Verification items for the finished model (mm, model axes). Face numbers are marked on the shaded views. A direction names the side the tool comes from. Give positions to 0.01 mm unless a question says otherwise; leave off trailing zeros. Write each loop counter-clockwise with the first axis right and the second up, starting at its lowest first coordinate (ties: lowest second). Pieces come first, ordered by that corner, then holes. Notation, with made-up numbers: (-1.5, 52) -> (17.5, 52) arc R3 cw to (17.5, 57) -> close; hole circle Ø1 at (-29.5, 65). An arc over 180 degrees is marked (long way). Answer as CSV lines item,"result". Start each with the question number.
1) Sectioned sample at B-B on z = 0. Record the cut outline in (x, y) (3 decimals), and give its area (3 significant figures).
2) Tool access check on the marked faces 1, 2 and 3. Record the directions out of +Z, -Z, +X, -X, +Y, -Y that give a thin tool (end or side, any length) a straight path to the whole face; none if there is none.
3) Mould release check, pull along X, two halves, no side actions. Record for the marked faces 4, 5 and 6: released by +X, released by -X, zero draft, split by the parting line, or undercut.
4) Sectioned sample at A-A on x = 0. Record the cut outline in (y, z) (3 decimals), and give its area (3 significant figures).
5) Sectioned sample at C-C on z = -9. Record the cut outline in (x, y).
6) Material ranges on L1, parallel to X at y = 0.7, z = 0 (3 decimals); L2, parallel to X at y = 3.25, z = 0 (3 decimals); L3, parallel to Z at x = 3.5, y = 3.25, recorded low to high.
7) Gauge pin test, flat ends, axial feed: pin 1 Ø2 at (x, z) = (1.5, 9) entering from +Y; pin 2 Ø1.5 at (y, z) = (2, -5.5) entering from -X; pin 3 Ø1 at (x, z) = (8.5, -1) entering from +Y; pin 4 Ø5 at (x, y) = (8.5, 9.5) entering from -Z. Record the tip position at first contact, or that the pin passes through.
8) Sectioned sample at D-D on y = 10.5. Record the cut outline in (x, z).
```python
from build123d import *


with BuildPart() as part:
    # Sketch1 → 20 and 58 (revolve)
    with BuildSketch(Plane.XY, mode=Mode.PRIVATE) as f_20_and_58_sk:
        Polygon((1.5, 14.9), (1.5, 0), (3.5, 0), (3.5, 1.2), (9.5, 1.2), (9.5, 0), (11.875, 0), (11.875, 4), (9.5, 4), (9.5, 3), (5.55, 3), (5.55, 14.9), align=None)
    revolve(f_20_and_58_sk.sketch.rotate(Axis((0, 0, 0), (0, 1, 0)), 90), axis=Axis((0, 0, 0), (0, 1, 0)))


solid = part.part
```
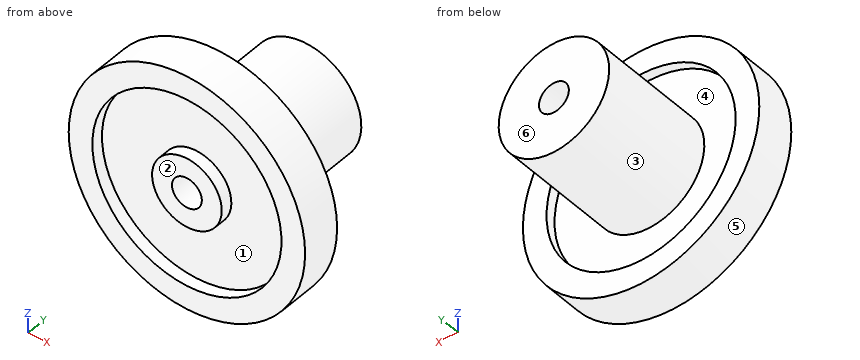
Ans:
1,outline,"(-11.875, 0) -> (-9.5, 0) -> (-9.5, 1.2) -> (-3.5, 1.2) -> (-3.5, 0) -> (-1.5, 0) -> (-1.5, 14.9) -> (-5.55, 14.9) -> (-5.55, 3) -> (-9.5, 3) -> (-9.5, 4) -> (-11.875, 4) -> close; (1.5, 0) -> (3.5, 0) -> (3.5, 1.2) -> (9.5, 1.2) -> (9.5, 0) -> (11.875, 0) -> (11.875, 4) -> (9.5, 4) -> (9.5, 3) -> (5.55, 3) -> (5.55, 14.9) -> (1.5, 14.9) -> close"
1,area,"149 mm²"
2,face 1,"-Y"
2,face 2,"+Z, -Z, +X, -X, -Y"
2,face 3,"+Y"
3,face 4,"undercut"
3,face 5,"split by the parting line"
3,face 6,"zero draft"
4,outline,"(0, -11.875) -> (4, -11.875) -> (4, -9.5) -> (3, -9.5) -> (3, -5.55) -> (14.9, -5.55) -> (14.9, -1.5) -> (0, -1.5) -> (0, -3.5) -> (1.2, -3.5) -> (1.2, -9.5) -> (0, -9.5) -> close; (0, 1.5) -> (14.9, 1.5) -> (14.9, 5.55) -> (3, 5.55) -> (3, 9.5) -> (4, 9.5) -> (4, 11.875) -> (0, 11.875) -> (0, 9.5) -> (1.2, 9.5) -> (1.2, 3.5) -> (0, 3.5) -> close"
4,area,"149 mm²"
5,outline,"(-7.75, 0) -> (-3.04, 0) -> (-3.04, 1.2) -> (3.04, 1.2) -> (3.04, 0) -> (7.75, 0) -> (7.75, 4) -> (3.04, 4) -> (3.04, 3) -> (-3.04, 3) -> (-3.04, 4) -> (-7.75, 4) -> close"
6,L1,"x = -11.875 to -9.5, -3.5 to -1.5, 1.5 to 3.5, 9.5 to 11.875"
6,L2,"x = -11.875 to -9.5, -5.55 to -1.5, 1.5 to 5.55, 9.5 to 11.875"
6,L3,"z = -11.35 to -8.83, -4.31 to 4.31, 8.83 to 11.35"
7,pin 1,"stops at y = 4"
7,pin 2,"stops at x = -10.88"
7,pin 3,"stops at y = 3"
7,pin 4,"passes through"
8,outline,"circle Ø11.1 at (0, 0); hole circle Ø3 at (0, 0)"
